Build history of the part. All positions in model axes, mm. Round coordinates to 2 decimals unless told otherwise and drop trailing zeros. Write each loop counter-clockwise with the first axis right and the second up, starting at its lowest first coordinate (ties: lowest second). Pieces come first, ordered by that corner, then holes. Notation, with made-up numbers: (73.25, -33.75) -> (109.25, -33.75) arc R8 cw to (109.25, -18.75) -> close; hole circle Ø8 at (86.5, 37.5). An arc over 180 degrees is marked (long way). Answer in a Markdown table with one row per item.
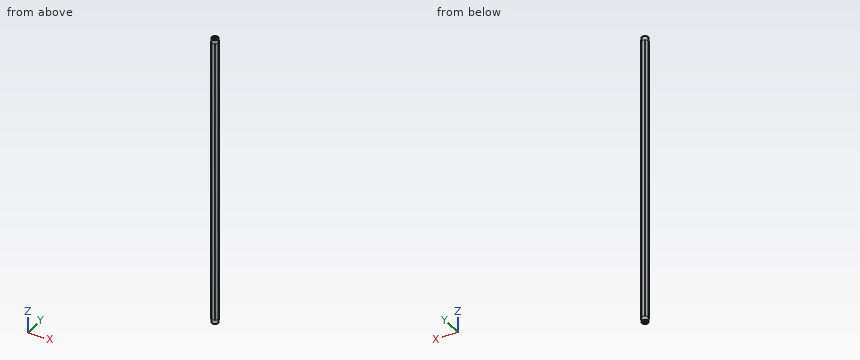
```python
from build123d import *

# Parameters (mm, degrees)
BOSS_EXTRUDE1_DEPTH = 292.1
SKETCH3_OUTSIDE_W   = 133.568
SKETCH3_OUTSIDE_H   = 131.604
SKETCH3_OUTSIDE_R   = 6.35
CUT_EXTRUDE2_DEPTH  = 7.9502
SKETCH4_OUTSIDE_W   = 133.568
SKETCH4_OUTSIDE_H   = 131.604
SKETCH4_OUTSIDE_R   = 6.858
CUT_EXTRUDE3_DEPTH  = 585.280519813
SKETCH5_R           = 2.4892
CUT_EXTRUDE4_DEPTH  = 585.274759564


with BuildPart() as part:
    # Sketch1 → Boss-Extrude1 (new, symmetric)
    with BuildSketch(Plane.XY):
        Polygon((7.332348419, 0), (3.666174209, 6.35), (-3.666174209, 6.35), (-7.332348419, 0), (-3.666174209, -6.35), (3.666174209, -6.35), align=None)
    extrude(amount=BOSS_EXTRUDE1_DEPTH, both=True)

    # Sketch3 outside → Cut-Extrude2 (cut)
    with BuildSketch(Plane.XY.offset(292.1)):
        Rectangle(SKETCH3_OUTSIDE_W, SKETCH3_OUTSIDE_H)
        Circle(SKETCH3_OUTSIDE_R, mode=Mode.SUBTRACT)
    cut_extrude2 = extrude(amount=-CUT_EXTRUDE2_DEPTH, mode=Mode.SUBTRACT)

    # Mirror1: Cut-Extrude2 across plane
    add(cut_extrude2.mirror(Plane.XY), mode=Mode.SUBTRACT)

    # Sketch4 outside → Cut-Extrude3 (cut, through all)
    with BuildSketch(Plane.XY.offset(292.1)):
        Rectangle(SKETCH4_OUTSIDE_W, SKETCH4_OUTSIDE_H)
        Circle(SKETCH4_OUTSIDE_R, mode=Mode.SUBTRACT)
    extrude(amount=-CUT_EXTRUDE3_DEPTH, mode=Mode.SUBTRACT)

    # Sketch5 → Cut-Extrude4 (cut, through all)
    with BuildSketch(Plane.XY.offset(292.1)):
        Circle(SKETCH5_R)
    extrude(amount=-CUT_EXTRUDE4_DEPTH, mode=Mode.SUBTRACT)


solid = part.part
```
Q1. Saw through at A-A on z = 187.5. Write the cut outline in (x, y).
A:
| item | result |
|---|---|
| outline | (-6.79, -0.93) -> (-4.2, -5.42) arc R6.86 ccw to (-2.59, -6.35) -> (2.59, -6.35) arc R6.86 ccw to (4.2, -5.42) -> (6.79, -0.93) arc R6.86 ccw to (6.79, 0.93) -> (4.2, 5.42) arc R6.86 ccw to (2.59, 6.35) -> (-2.59, 6.35) arc R6.86 ccw to (-4.2, 5.42) -> (-6.79, 0.93) arc R6.86 ccw to start; hole circle Ø4.98 at (0, 0) |
Q2. Drop a flat-ended pin along its axis: P1, Ø3, axis at y = 4, z = -174.5, coming from the -X side. Give the stop position or say it passes through.
A:
| item | result |
|---|---|
| P1 | x = -5.89 |
Q3. Wall check: line 1 (Y direction, x = -0.75, z = 256.5); line 2 (X direction, y = 2, z = 90.5); line 3 (X direction, y = -3, z = 249.5). Give the ranges that are in metal, low to high. Write a range as [from, to].
A:
| item | result |
|---|---|
| line 1 | [-6.35, -2.37], [2.37, 6.35] |
| line 2 | [-6.18, -1.48], [1.48, 6.18] |
| line 3 | [-5.6, 5.6] |
